```python
from build123d import *

# Parameters (mm, degrees)
SKETCH1_W                  = 111
SKETCH1_H                  = 100
BOSS_EXTRUDE1_DEPTH        = 3
F_3_5_3_5_DIAMETER_HOLE1_D = 3.5


with BuildPart() as part:
    # Sketch1 → Boss-Extrude1 (new body)
    with BuildSketch(Plane.XY):
        with Locations((-54, -41)):
            Rectangle(SKETCH1_W, SKETCH1_H)
    extrude(amount=BOSS_EXTRUDE1_DEPTH)

    # Ø3.5 (3.5) Diameter Hole1 (through all)
    with Locations(Plane.XY.offset(3)):
        with Locations((0, 0), (-108, 0), (-93, -82), (0, -60)):
            Hole(F_3_5_3_5_DIAMETER_HOLE1_D / 2)


solid = part.part
```
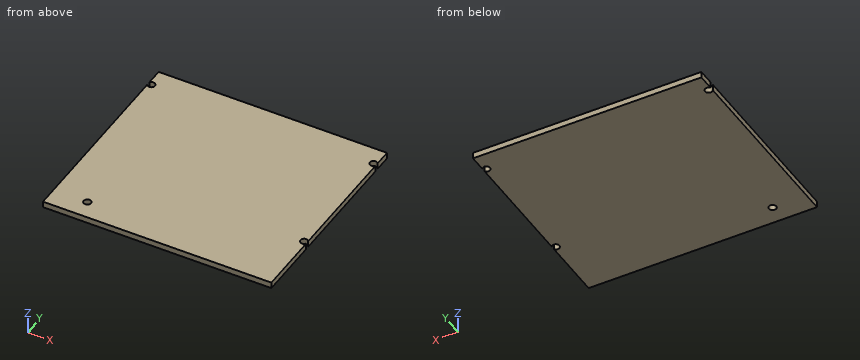
Model file for the job. Use its own axes, mm. Coordinates: 2 decimals unless noted, no trailing zeros. Order: outer loops, then holes, each group sorted by start corner. A loop starts at its lowest first (then second) coordinate and runs counter-clockwise, first axis right, second up. Notation, with made-up numbers: (78.5, 63.25) - (126.5, 63.25) arc R13 ccw to (126.5, 67.25) - close; hole circle Ø2 at (-22, 34.25). An arc over 180 degrees is marked (long way). Return JSON: item names as keys, results as strings. Group by question number.
1) Saw through at A-A, the plane x = -93. Write the cut outline in (y, z).
2) Flat gauge pin, fed straight in: P1, Ø3, axis at x = -108, y = 0, coming from the +Z side. Where does the tip first touch, or does it go through?
3) Probe line 1 (Y direction, x = 0, z = 0.7); line 2 (Y direction, x = -93, z = 1.3); line 3 (X direction, y = -82, z = 2.4). List the from-to ranges inside material, lowest first. Write a range as from..to.
4) Saw through at B-B, the plane x = 0. Write the cut outline in (y, z).
Values found:
{
 "1": {"outline": "(-91, 0) - (-83.75, 0) - (-83.75, 3) - (-91, 3) - close; (-80.25, 0) - (9, 0) - (9, 3) - (-80.25, 3) - close"},
 "2": {"P1": "passes through"},
 "3": {"line 1": "y = -91..-61.75, -58.25..-1.75, 1.75..9", "line 2": "y = -91..-83.75, -80.25..9", "line 3": "x = -109.5..-94.75, -91.25..1.5"},
 "4": {"outline": "(-91, 0) - (-61.75, 0) - (-61.75, 3) - (-91, 3) - close; (-58.25, 0) - (-1.75, 0) - (-1.75, 3) - (-58.25, 3) - close; (1.75, 0) - (9, 0) - (9, 3) - (1.75, 3) - close"}
}
